For this review, take the finished solid that the model builds, in its own axes (mm). A direction names the side the tool comes from. Give positions to 0.01 mm unless a question says otherwise; leave off trailing zeros. Loops run counter-clockwise (first coordinate to the right, second up) from the corner with the lowest first, then second, coordinate; pieces in that order, holes last. Notation, with made-up numbers: (66.5, 68) - (73.5, 68) arc R33 ccw to (73.5, 98) - close; hole circle Ø4 at (10.5, 9.25). An arc over 180 degrees is marked (long way). Answer as CSV lines item,"result".
from build123d import *

# Parameters (mm, degrees)
BOSS_EXTRUDE2_DEPTH = 15
CUT_EXTRUDE2_DEPTH  = 15
SKETCH5_W           = 50
SKETCH5_H           = 70
BOSS_EXTRUDE3_DEPTH = 10
SKETCH6_W           = 40
SKETCH6_H           = 25
BOSS_EXTRUDE4_DEPTH = 50
RIB1_REACH          = 95.575
SKETCH10_WALL_W     = 217.43394397
SKETCH10_WALL_H     = 10
SKETCH11_R          = 15
CUT_EXTRUDE3_DEPTH  = 25


with BuildPart() as part:
    # Sketch2 → Boss-Extrude2 (new body)
    with BuildSketch(Plane.XY):
        with BuildLine():
            Line((-25, 37.5), (-25, -37.5))
            Line((-25, -37.5), (25, -37.5))
            Line((25, -37.5), (25, 37.5))
            ThreePointArc((25, 37.5), (0, 62.5), (-25, 37.5))
        make_face()
    extrude(amount=BOSS_EXTRUDE2_DEPTH)

    # Sketch4 → Cut-Extrude2 (cut)
    with BuildSketch(Plane.XY.offset(15)):
        with BuildLine():
            Line((-15, 37.5), (15, 37.5))
            ThreePointArc((15, 37.5), (0, 52.5), (-15, 37.5))
        make_face()
    extrude(amount=-CUT_EXTRUDE2_DEPTH, mode=Mode.SUBTRACT)

    # Sketch5 → Boss-Extrude3 (add)
    with BuildSketch(Plane.XY.offset(15)):
        with Locations((0, -2.5)):
            Rectangle(SKETCH5_W, SKETCH5_H)
    extrude(amount=BOSS_EXTRUDE3_DEPTH)

    # Sketch6 → Boss-Extrude4 (add)
    with BuildSketch(Plane.ZY.offset(25)):
        with Locations((45, 0)):
            Rectangle(SKETCH6_W, SKETCH6_H)
    extrude(amount=-BOSS_EXTRUDE4_DEPTH)

    # Sketch10 wall → Rib1 (add, up to next)
    with BuildSketch(Plane(origin=(0, 22.5, 35), x_dir=(0, -0.707106781187, 0.707106781187), z_dir=(0, -0.707106781187, -0.707106781187)), mode=Mode.PRIVATE) as rib1_sk1:
        Rectangle(SKETCH10_WALL_W, SKETCH10_WALL_H)
    rib1_tool1 = extrude(rib1_sk1.sketch, amount=RIB1_REACH, mode=Mode.PRIVATE) - part.part
    add(rib1_tool1.solids().sort_by_distance((0, 22.5, 35))[0])

    # Sketch11 → Cut-Extrude3 (cut)
    with BuildSketch(Plane(origin=(0, 12.5, 0), x_dir=(1, 0, 0), z_dir=(0, 1, 0))):
        with Locations((0, -65)):
            Circle(SKETCH11_R)
    extrude(amount=-CUT_EXTRUDE3_DEPTH, mode=Mode.SUBTRACT)


solid = part.part
1) Machinability: for faces 1 (the flat face through (-6, 12.5, 45)), 2 (the flat face through (15, 23, 25)), 3 (the flat face through (0, -12.5, 40)), which of the approach directions +Z, -Z, +X, -X, +Y, -Y give a long, thin tool a straight path to every point of the face, cutting with its end or side? Answer none if there is none.
From the geometry:
face 1,"+Z, +Y"
face 2,"+Z, +X, +Y"
face 3,"+Z, +X, -X, -Y"
2) Wall thickness on line 1 (Y direction, x = -8, z = 21); line 2 (Z direction, x = 0.5, y = 9.5); line 3 (Y direction, x = 19.5, z = 39.5): over which ranges is each line inside the solid? List them lowest first. Write a range as from..to.
From the geometry:
line 1,"y = -37.5..32.5"
line 2,"z = 0..50.01"
line 3,"y = -12.5..12.5"
3) Consider section B-B on z = 26.5. Write out the cut boundary in (x, y), and give its area (4 significant figures).
From the geometry:
outline,"(-25, -12.5) - (25, -12.5) - (25, 12.5) - (5, 12.5) - (5, 31) - (-5, 31) - (-5, 12.5) - (-25, 12.5) - close"
area,"1,435 mm^2"
4) Insertion check: P1, Ø5, axis at x = 16.5, y = -15.5, coming from the +Z side; P2, Ø9, axis at x = -3, y = 43, coming from the +Z side; P3, Ø20, axis at x = -2, z = 45.5, coming from the +Y side; P4, Ø4.5, axis at x = 6, z = 8, coming from the +Y side. Each pin has a flat end and moves straight along its axis. Give the tip position at first contact, or say it passes through.
From the geometry:
P1,"stops at z = 25"
P2,"passes through"
P3,"stops at y = 22"
P4,"stops at y = 62.22"
5) Draft analysis for pull direction Y (two halves, no side actions). For faces 4 (the flat face through (0, -25, 25)), 5 (the flat face through (-0.1, 22.6, 34.9)), 6 (the cylindrical face through (0.33, 52.496, 7.605)), state which applies: pulls with the +Y half, pulls with the -Y half, needs draft (parallel to the pull), parting line crosses it, or undercut.
From the geometry:
face 4,"needs draft"
face 5,"pulls with the +Y half"
face 6,"undercut"
6) Consider section C-C on y = 22. Write out the cut boundary in (x, z).
From the geometry:
outline,"(-25, 0) - (25, 0) - (25, 25) - (5, 25) - (5, 35.5) - (-5, 35.5) - (-5, 25) - (-25, 25) - close"
7) Consider section D-D on x = -20. Write out the cut boundary in (y, z), and give its area (3 significant figures).
From the geometry:
outline,"(-37.5, 0) - (52.5, 0) - (52.5, 15) - (32.5, 15) - (32.5, 25) - (12.5, 25) - (12.5, 65) - (-12.5, 65) - (-12.5, 25) - (-37.5, 25) - close"
area,"3,050 mm^2"
8) Consider section A-A on x = 0. Write out the cut boundary in (y, z), and give its area (3 significant figures).
From the geometry:
outline,"(-37.5, 0) - (37.5, 0) - (37.5, 15) - (32.5, 15) - (32.5, 25) - (12.5, 45) - (12.5, 50) - (-12.5, 50) - (-12.5, 25) - (-37.5, 25) - close; (52.5, 0) - (62.5, 0) - (62.5, 15) - (52.5, 15) - close"
area,"2,800 mm^2"
